Check sheet for the drawn part. Datum: minimum x, y, z corner. Units: mm. A direction names the side the tool comes from. Round coordinates to 2 decimals unless told otherwise and drop trailing zeros. Order: outer loops, then holes, each group sorted by start corner. A loop starts at its lowest first (then second) coordinate and runs counter-clockwise, first axis right, second up. Notation, with made-up numbers: (-38.5, -18.75) -> (-3.5, -18.75) arc R13 ccw to (-3.5, -10.75) -> close; hole circle Ø2 at (76.5, 64.25). An arc over 180 degrees is marked (long way). Answer as a JSON object with one key per item and string values. Group by question number.
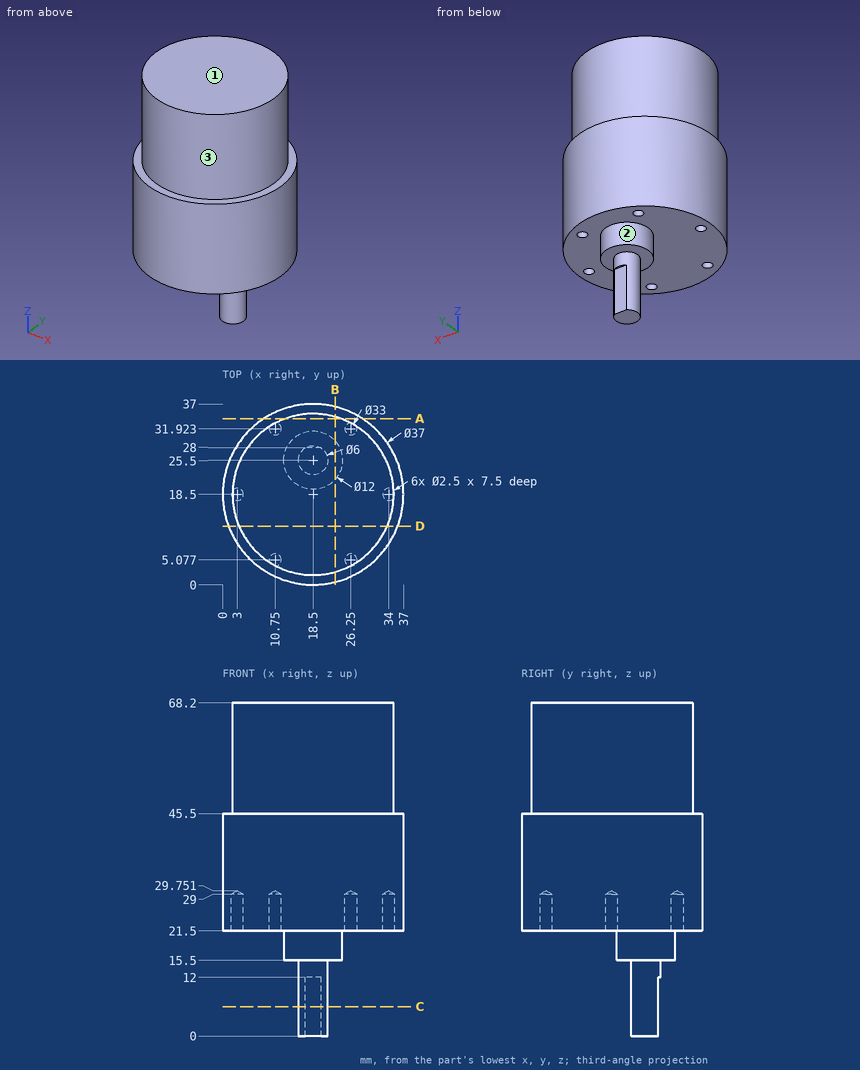
Item 1: Sectioned sample at D-D, the plane y = 12. Enter the section's corners in (x, z) (1 decimal).
Item 2: Sectioned sample at A-A, the plane y = 34. Enter the section's corners in (x, z).
Item 3: Depth check by flat-ended pin: pin 1 Ø10 at (x, y) = (29, 32) entering from -Z; pin 2 Ø2 at (x, y) = (26.25, 31.92) entering from -Z; pin 3 Ø3 at (x, z) = (26.5, 56.5) entering from -Y (1 decimal); pin 4 Ø12 at (x, z) = (4, 8.5) entering from +Y. Enter the tip coordinate at first touch or a pass-through.
Item 4: Set-up check for the marked faces 1, 2 and 3: record each of +Z, -Z, +X, -X, +Y, -Y from which the full face is reachable in a straight line by a thin tool's end or side.
Item 5: Sectioned sample at B-B, the plane x = 23. Enter the section's corners in (y, z) (1 decimal).
Item 6: Thickness scan on L1, parallel to Y at x = 26.25, z = 24.5; L2, parallel to Z at x = 5.5, y = 25.5; L3, parallel to Z at x = 17, y = 29. Record the ranges inside material, lowest first.
Item 7: Sectioned sample at C-C, the plane z = 6. Enter the section's corners in (x, y).
Result:
{
 "1": {"outline": "(1.2, 21.5) -> (35.8, 21.5) -> (35.8, 45.5) -> (33.7, 45.5) -> (33.7, 68.2) -> (3.3, 68.2) -> (3.3, 45.5) -> (1.2, 45.5) -> close"},
 "2": {"outline": "(8.4, 21.5) -> (28.6, 21.5) -> (28.6, 45.5) -> (24.16, 45.5) -> (24.16, 68.2) -> (12.84, 68.2) -> (12.84, 45.5) -> (8.4, 45.5) -> close"},
 "3": {"pin 1": "stops at z = 21.5", "pin 2": "stops at z = 29.15", "pin 3": "stops at y = 3.3", "pin 4": "passes through"},
 "4": {"face 1": "+Z, +X, -X, +Y, -Y", "face 2": "-Z", "face 3": "+Z"},
 "5": {"outline": "(0.6, 21.5) -> (21.5, 21.5) -> (21.5, 15.5) -> (29.5, 15.5) -> (29.5, 21.5) -> (36.4, 21.5) -> (36.4, 45.5) -> (34.4, 45.5) -> (34.4, 68.2) -> (2.6, 68.2) -> (2.6, 45.5) -> (0.6, 45.5) -> close"},
 "6": {"L1": "y = 1.7 to 3.83, 6.33 to 30.67, 33.17 to 35.3", "L2": "z = 21.5 to 68.2", "L3": "z = 15.5 to 68.2"},
 "7": {"outline": "(16.84, 28) arc R3 ccw (long way) to (20.16, 28) -> close"}
}
